The model under review builds one solid part; all positions refer to its coordinate system, in mm. Round coordinates to 2 decimals unless told otherwise and drop trailing zeros. Write each loop counter-clockwise with the first axis right and the second up, starting at its lowest first coordinate (ties: lowest second). Pieces come first, ordered by that corner, then holes.
Item 1: Add section A-A (y = 0). Give the boundary of the cut face in (x, z), plus the area to 3 significant figures.
Item 2: Add section B-B (z = -90.5). Give the boundary of the cut face in (x, y).
Item 3: To check wall thickness, follow L1, parallel to X at y = -0.1, z = -37; L2, parallel to X at y = -0.25, z = -74; L3, parallel to Z at x = -0.75, y = 0.3. State the ranges of each line that lie inside material, in increasing order.
Autodesk Inventor part; units mm, degrees
ref_plane "YZ Plane" through (0, 0, 0) normal (1, 0, 0) x (0, 1, 0)
ref_plane "XZ Plane" through (0, 0, 0) normal (0, 1, 0) x (-1, 0, 0)
ref_plane "XY Plane" through (0, 0, 0) normal (0, 0, 1) x (1, 0, 0)
sketch "Sketch5" plane through (0, 0, 0) normal (0, 0, 1) x (1, 0, 0)
  circle A0 centre (3, 0) radius 0.5
  line L0 (0, -0.7) -> (0, 0.7)
  point P0 (0, 0)
  dimension "d8" = 1
  dimension "d9" = 3
revolve "Revolution1" add sketch "Sketch5" angle 180 about axis through (0, -10, 0) along (0, -1, 0)
sketch "Sketch6" plane through (3, 0, 0) normal (0, 0, -1) x (-1, 0, 0)
  circle A0 centre (0, 0) radius 0.5
  circle A1 centre (6, 0) radius 0.5
  point P0 (3, 0)
extrude "Extrusion1" add sketch "Sketch6" along normal blind 100
sketch "Sketch7" plane through (3, 0, -100) normal (0, 0, -1) x (-1, 0, 0)
  circle A0 centre (0, 0) radius 0.5
  line L0 (3, -0.7) -> (3, 0.7)
  point P0 (3, 0)
revolve "Revolution2" add sketch "Sketch7" angle 180 about axis through (0, -10, -100) along (0, 1, 0)
properties part number "Rope"
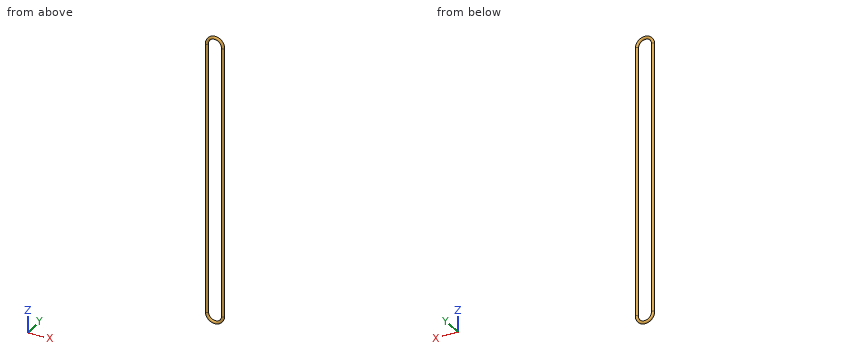
Numbers:
1. outline: (-3.5, -100) arc R3.5 ccw to (3.5, -100) - (3.5, 0) arc R3.5 ccw to (-3.5, 0) - close; hole (-2.5, -100) arc R2.5 ccw to (2.5, -100) - (2.5, 0) arc R2.5 ccw to (-2.5, 0) - close
1. area: 219 mm2
2. outline: circle Ø1 at (-3, 0); circle Ø1 at (3, 0)
3. L1: x = -3.49 to -2.51, 2.51 to 3.49
3. L2: x = -3.43 to -2.57, 2.57 to 3.43
3. L3: z = -103.32 to -102.49, 2.49 to 3.32
